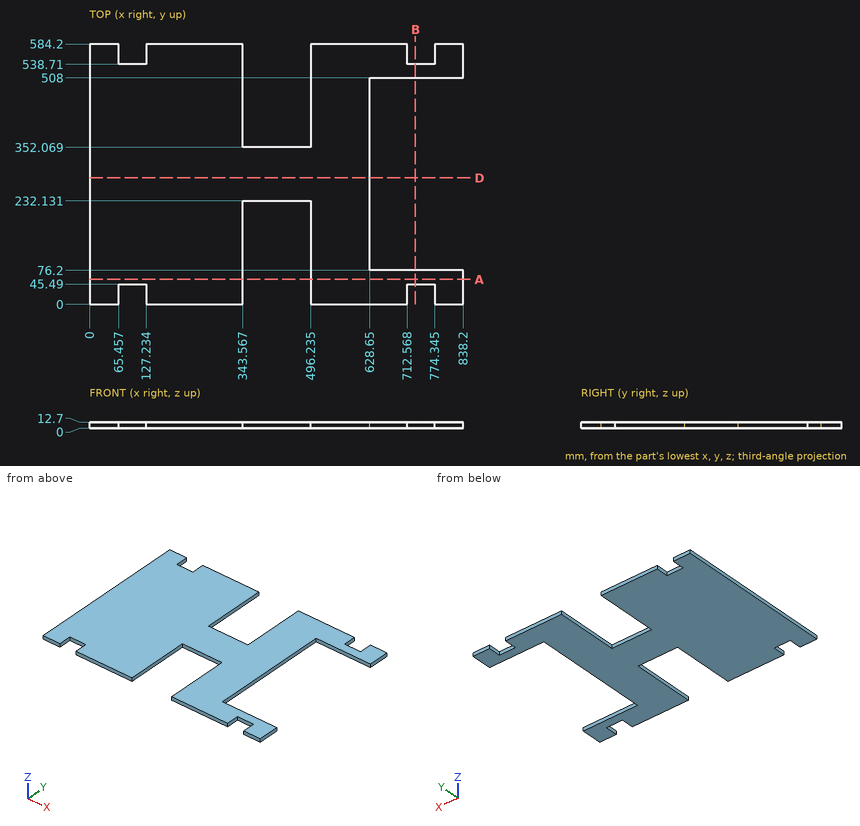
Print and shaded views of the part. All mm, measured from the part's lowest x, y and z. Give positions to 0.01 mm unless a question says otherwise; leave off trailing zeros. Order: outer loops, then holes, each group sorted by start corner. A loop starts at its lowest first (then second) coordinate and runs counter-clockwise, first axis right, second up. Notation, with made-up numbers: (61.25, -0.5) - (112.25, -0.5) arc R28 cw to (112.25, 20.5) - close; hole circle Ø1 at (-31, 33.25). An arc over 180 degrees is marked (long way). Use a Markdown table: item, result.
1) Probe L1, parallel to X at y = 70, z = 4.75 (1 decimal); L2, parallel to Y at x = 754, z = 8.5; L3, parallel to Y at x = 425, z = 9.75. List the from-to ranges inside material, lowest first. Write a range as from..to.
Checked values:
| item | result |
|---|---|
| L1 | 0..343.6, 496.2..838.2 |
| L2 | 45.49..76.2, 508..538.71 |
| L3 | 232.13..352.07 |
2) Saw through at D-D on y = 284. List the corners of the cut face in (x, z).
Checked values:
| item | result |
|---|---|
| outline | (0, 0) - (628.65, 0) - (628.65, 12.7) - (0, 12.7) - close |
3) Saw through at B-B on x = 731. List the corners of the cut face in (y, z).
Checked values:
| item | result |
|---|---|
| outline | (45.49, 0) - (76.2, 0) - (76.2, 12.7) - (45.49, 12.7) - close; (508, 0) - (538.71, 0) - (538.71, 12.7) - (508, 12.7) - close |
4) Flat gauge pins, fed straight in: P1, Ø6.5, axis at x = 110, z = 5.5, coming from the +Y side; P2, Ø4, axis at x = 426.5, z = 4.5, coming from the +Y side; P3, Ø1.5, axis at y = 137.5, z = 7.5, coming from the +X side; P4, Ø4, axis at y = 332, z = 3, coming from the -X side. Where does each tip first touch, or does it go through?
Checked values:
| item | result |
|---|---|
| P1 | y = 538.71 |
| P2 | y = 352.07 |
| P3 | x = 628.65 |
| P4 | x = 0 |
5) Saw through at A-A on y = 56. List the corners of the cut face in (x, z) (1 decimal).
Checked values:
| item | result |
|---|---|
| outline | (0, 0) - (343.6, 0) - (343.6, 12.7) - (0, 12.7) - close; (496.2, 0) - (838.2, 0) - (838.2, 12.7) - (496.2, 12.7) - close |
